Could you check a few things on this model? Use its own coordinates, in mm. A direction names the side the tool comes from. Coordinates: 2 decimals unless noted, no trailing zeros. Loops run counter-clockwise (first coordinate to the right, second up) from the corner with the lowest first, then second, coordinate; pieces in that order, holes last. Notation, with made-up numbers: (40, 62) -> (80, 62) arc R31 ccw to (80, 100) -> close; hole circle Ø10 at (-24, -31.5). An arc over 180 degrees is marked (long way). One line per question, with ' | ' between items.
from build123d import *

# Parameters (mm, degrees)
PAD003_DEPTH = 32
SKETCH_W     = 15
SKETCH_H     = 4.7
PAD_DEPTH    = 32


with BuildPart() as part:
    # Sketch005 → Pad003 (new body)
    with BuildSketch(Plane.XY):
        Polygon((-2.5, 9.85), (2.5, 9.85), (2.5, -9.85), (-2.5, -9.85), (-5.5, -9.85), (-5.5, -6.15), (-2.5, -6.15), (-2.5, 6.15), (-5.5, 6.15), (-5.5, 9.85), align=None)
    extrude(amount=PAD003_DEPTH)

    # Sketch → Pad (join)
    with BuildSketch(Plane.XY):
        with Locations((10, 0)):
            Rectangle(SKETCH_W, SKETCH_H)
    extrude(amount=PAD_DEPTH)


solid = part.part
1) I need wall thicknesses on line 1 along Y through (x, z) = (7, 30.5); line 2 along X through (y, z) = (-7, 4); line 3 along X through (y, z) = (1, 22). Which ranges of each line are inside material? Lowest first, please. Write a range as from..to.
Data:
line 1: -2.35..2.35 | line 2: -5.5..2.5 | line 3: -2.5..17.5
2) I'm going to push flat-ended pins straight in: pin 1 Ø2 at (y, z) = (-7.5, 11) entering from +X; pin 2 Ø1 at (x, z) = (12.5, 11.5) entering from +Y; pin 3 Ø5 at (y, z) = (-1.5, 6.5) entering from -X. Where does each tip first touch, or does it pass through?
Data:
pin 1: x = 2.5 | pin 2: y = 2.35 | pin 3: x = -2.5
3) If we section it at A-A on x = -3.75: Please give me the cut outline in (y, z), and give its area (3 significant figures).
Data:
outline: (-9.85, 0) -> (-6.15, 0) -> (-6.15, 32) -> (-9.85, 32) -> close; (6.15, 0) -> (9.85, 0) -> (9.85, 32) -> (6.15, 32) -> close | area: 237 mm²
4) If we section it at B-B on z = 27: Please give me the cut outline in (x, y).
Data:
outline: (-5.5, -9.85) -> (2.5, -9.85) -> (2.5, -2.35) -> (17.5, -2.35) -> (17.5, 2.35) -> (2.5, 2.35) -> (2.5, 9.85) -> (-5.5, 9.85) -> (-5.5, 6.15) -> (-2.5, 6.15) -> (-2.5, -6.15) -> (-5.5, -6.15) -> close
5) If we section it at D-D on x = 14: Please give me the cut outline in (y, z).
Data:
outline: (-2.35, 0) -> (2.35, 0) -> (2.35, 32) -> (-2.35, 32) -> close
6) If we section it at C-C on y = -4.75: Please give me the cut outline in (x, z).
Data:
outline: (-2.5, 0) -> (2.5, 0) -> (2.5, 32) -> (-2.5, 32) -> close
7) We'd pull the mould along Y, two halves only. Please class faces 6 (the face through (-1, 9.85, 16)), 7 (the face through (-2.5, 0, 16)), 8 (the face through (-5.5, -8, 16)): pulls with the +Y half, pulls with the -Y half, needs draft (parallel to the pull), parting line crosses it, or undercut.
Data:
face 6: pulls with the +Y half | face 7: undercut | face 8: needs draft
8) On a 3-axis mill with a long thin cutter (end or side, diameter ignored), from which of +Z, -Z, +X, -X, +Y, -Y can I reach the whole of each face in a straight line? I mean faces 1 (the face through (17.5, 0, 16)), 2 (the face through (2.5, 6, 16)), 3 (the face through (-4, -6.15, 16)), 4 (the face through (4, 0, 0)), 5 (the face through (2.5, -6, 16)). Say none if no direction works.
Data:
face 1: +Z, -Z, +X, +Y, -Y | face 2: +Z, -Z, +X, +Y | face 3: +Z, -Z, -X | face 4: -Z, +X, -X, +Y, -Y | face 5: +Z, -Z, +X, -Y
